```python
from build123d import *

# Parameters (mm, degrees)
F2_R    = 1.99999
F3_SIZE = 0.99999


# Not quite as in the source:
# - a fillet or chamfer is up to 0.001 mm smaller than in the source, because OpenCascade refuses the exact size


with BuildPart() as f1:
    # F0 (on Top) → F1 (revolve)
    with BuildSketch(Plane.XY):
        Polygon((-24.5, 0), (-24.5, 14.3020306939), (-24.5, 15), (-25.5, 15), (-25.5, 5), (-27.5, 5), (-27.5, 15), (-29.5, 15), (-29.5, 0), align=None)
    revolve(axis=Axis((0, 7.5544440188, 0), (0, -1, 0)))

    # F2 (radius 2 in the source; OpenCascade refuses exactly that, so slightly less here)
    f2_edges = [f1.edges().sort_by_distance(p)[0] for p in [
        (29.5, 15, 0),
        (29.5, 0, 0),
    ]]
    fillet(f2_edges, radius=F2_R)

    # F3 (size 1 in the source; OpenCascade refuses exactly that, so slightly less here)
    f3_edges = [f1.edges().sort_by_distance(p)[0] for p in [
        (24.5, 15, 0),
    ]]
    chamfer(f3_edges, length=F3_SIZE)


solid = f1.part
```
Work out the finished part from the listing and answer in its coordinate system (mm). Coordinates: 2 decimals unless noted, no trailing zeros. Order: outer loops, then holes, each group sorted by start corner. A loop starts at its lowest first (then second) coordinate and runs counter-clockwise, first axis right, second up. Notation, with made-up numbers: (57.25, -14) - (113.25, -14) arc R23 ccw to (113.25, 10) - close; hole circle Ø9 at (9, -10). An arc over 180 degrees is marked (long way). Answer as a JSON object with one key per item and string values.
1. Each of these flat-tipped pins is pushed along its axis until it touches: P1, Ø3, axis at x = -14.5, z = 20, coming from the -Y side; P2, Ø2, axis at y = 8.5, z = -15.5, coming from the +X side; P3, Ø6, axis at y = 8.5, z = -8.5, coming from the -X side; P4, Ø1.5, axis at x = 20, y = 7, coming from the +Z side. Where does it stop, or does it pass through?
Output values:
{"P1": "stops at y = 0", "P2": "stops at x = 25.69", "P3": "stops at x = -28.98", "P4": "stops at z = 22.35"}
2. Find section B-B on y = 11. Determine the outline of the cut face in (x, z).
Output values:
{"outline": "circle Ø59 at (0, 0); circle Ø51 at (0, 0); hole circle Ø55 at (0, 0); hole circle Ø49 at (0, 0)"}
3. The mould has two halves that part along Z. Classify faces 1 (the face through (-13.17, 7.1, -20.66)), 2 (the face through (-28.14, 7.42, -8.86)), 3 (the face through (18.2, 5, 18.2)), 4 (the face through (25, 0, 2)): +Z half, -Z half, draft (parallel to the pull), parting line (faces both ways), or undercut.
Output values:
{"face 1": "undercut", "face 2": "parting line", "face 3": "undercut", "face 4": "draft"}
4. Consider line 1 (X direction, y = 7.5, z = 0); line 2 (Z direction, x = -3, y = 8.25). Determine where each line is inside the solid, lowest interval first.
Output values:
{"line 1": "x = -29.5 to -27.5, -25.5 to -24.5, 24.5 to 25.5, 27.5 to 29.5", "line 2": "z = -29.35 to -27.34, -25.32 to -24.32, 24.32 to 25.32, 27.34 to 29.35"}
